Here's the drawing with two shaded views (mm, measured from the low corner). I have some questions. Round coordinates to 2 decimals unless told otherwise and drop trailing zeros. Loops run counter-clockwise (first coordinate to the right, second up) from the corner with the lowest first, then second, coordinate; pieces in that order, holes last.
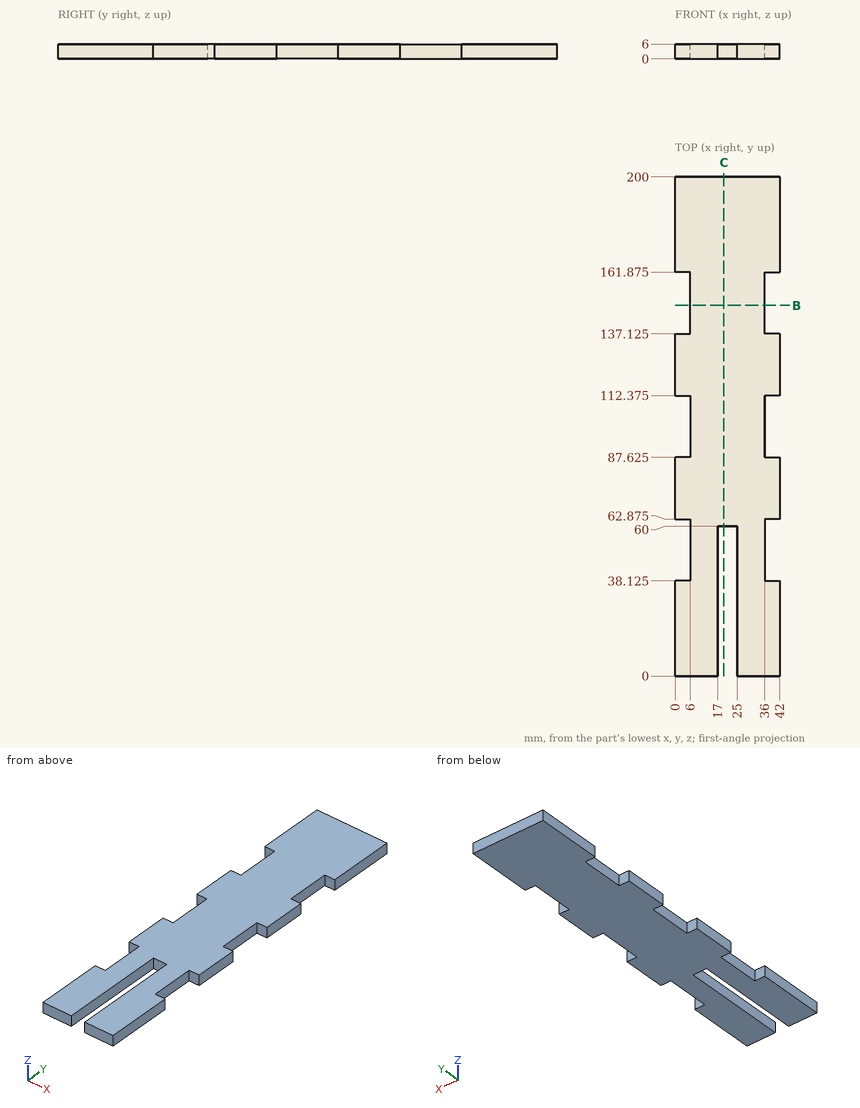
(1) If we section it at B-B, the plane y = 148.5: List the corners of the cut face in (x, z) for me, then the cut area to 3 significant figures.
Worked answers:
outline: (6, 0) - (36, 0) - (36, 6) - (6, 6) - close
area: 180 mm2
(2) If we section it at C-C, the plane x = 19.5: List the corners of the cut face in (y, z) for me.
Worked answers:
outline: (60, 0) - (200, 0) - (200, 6) - (60, 6) - close
(3) If I drill on line 1 (Y direction, x = 5, z = 1.4) (3 decimals); line 2 (X direction, y = 54, z = 3.55); line 3 (X direction, y = 19, z = 4.1), over which ranges is the centre line in solid material (lowest first)?
Worked answers:
line 1: y = 0 to 38.125, 62.875 to 87.625, 112.375 to 137.125, 161.875 to 200
line 2: x = 6 to 17, 25 to 36
line 3: x = 0 to 17, 25 to 42
